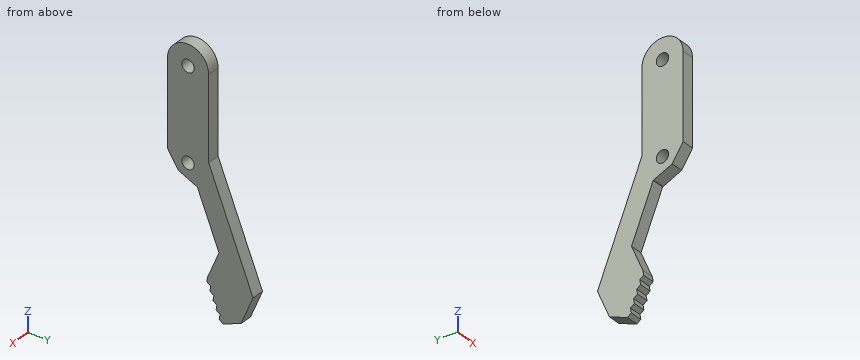
from build123d import *

# Parameters (mm, degrees)
SKETCH1_R             = 5
SKETCH1_R_2           = 1.5
BOSS_EXTRUDE1_DEPTH   = 3
BOSS_EXTRUDE2_START   = -3
BOSS_EXTRUDE2_DEPTH   = 3
CUT_EXTRUDE2_DEPTH    = 65.81382707
CORTAR_EXTRUIR1_DEPTH = 3
SCALE1_SCALE          = 0.888888889


# Read off the part's stored shape, not the designer's step: Cortar-Extruir1
with BuildPart() as part:
    # Sketch1 → Boss-Extrude1 (new body)
    # profile 1 of 3: a face of its own
    with BuildSketch(Plane(origin=(0, 0, 0), x_dir=(0, 0, -1), z_dir=(1, 0, 0))):
        with Locations((5, 5)):
            Circle(SKETCH1_R)
        with Locations((5, 5)):
            Circle(SKETCH1_R_2, mode=Mode.SUBTRACT)
    # profile 2 of 3: a face of its own
    with BuildSketch(Plane(origin=(0, 0, 0), x_dir=(0, 0, -1), z_dir=(1, 0, 0))):
        with BuildLine():
            ThreePointArc((10, 5), (8.535533906, 1.464466094), (5, 0))
            Line((5, 0), (27, 0))
            ThreePointArc((27, 0), (22, 5), (27, 10))
            Line((27, 10), (5, 10))
            ThreePointArc((5, 10), (8.535533906, 8.535533906), (10, 5))
        make_face()
    # profile 3 of 3: a face of its own
    with BuildSketch(Plane(origin=(0, 0, 0), x_dir=(0, 0, -1), z_dir=(1, 0, 0))):
        with Locations((27, 5)):
            Circle(SKETCH1_R)
        with Locations((27, 5)):
            Circle(SKETCH1_R_2, mode=Mode.SUBTRACT)
    extrude(amount=BOSS_EXTRUDE1_DEPTH)

    # Sketch2 → Boss-Extrude2 (add)
    with BuildSketch(Plane(origin=(3, 0, 0), x_dir=(0, 0, -1), z_dir=(1, 0, 0)).offset(BOSS_EXTRUDE2_START)):
        with BuildLine():
            ThreePointArc((27, 10), (29.694507461, 9.21184396), (31.53953799, 7.095851816))
            Line((31.53953799, 7.095851816), (31.610157793, 7.262674791))
            Line((31.610157793, 7.262674791), (44.585599673, 12.519851602))
            Line((44.585599673, 12.519851602), (51.097249205, 9.763328363))
            Line((51.097249205, 9.763328363), (60.365421977, 13.518454657))
            Line((60.365421977, 13.518454657), (56.610295683, 22.786627428))
            Line((56.610295683, 22.786627428), (25.051124858, 10))
            Line((25.051124858, 10), (27, 10))
        make_face()
        Polygon((60.365421977, 13.518454657), (51.097249205, 9.763328363), (51.333822162, 9.179433479), (60.601994933, 12.934559772), align=None)
    extrude(amount=BOSS_EXTRUDE2_DEPTH)

    # Sketch4 → Cut-Extrude2 (cut, through all)
    with BuildSketch(Plane(origin=(3, 0, 0), x_dir=(0, 0, -1), z_dir=(1, 0, 0))):
        Polygon((56.610295683, 22.786627428), (51.684261855, 20.790777803), (58.606145308, 17.8605936), align=None)
    extrude(amount=-CUT_EXTRUDE2_DEPTH, mode=Mode.SUBTRACT)

    # Cortar-Extruir1 outline → Cortar-Extruir1 (cut)
    with BuildSketch(Plane.YZ):
        with BuildLine():
            ThreePointArc((0, -27), (2.305492538, -31.21184396), (7.095851816, -31.53953799))
            Line((7.095851816, -31.53953799), (2.664871714, -29.583874941))
            Line((2.664871714, -29.583874941), (0, -25.53953799))
            Line((0, -25.53953799), (0, -27))
        make_face()
        Polygon((13.518454657, -60.365421977), (12.559047143, -59.675177656), (12.934559772, -60.601994933), align=None)
        Polygon((12.767429398, -58.511787422), (11.808021884, -57.821543102), (12.559047143, -59.675177656), align=None)
        Polygon((12.01640414, -56.658152868), (11.056996626, -55.967908548), (11.808021884, -57.821543102), align=None)
        Polygon((11.265378881, -54.804518314), (10.305971367, -54.114273993), (11.056996626, -55.967908548), align=None)
        Polygon((10.514353622, -52.95088376), (9.554946108, -52.260639439), (10.305971367, -54.114273993), align=None)
        Polygon((9.554946108, -52.260639439), (9.763328363, -51.097249205), (9.179433479, -51.333822162), align=None)
    extrude(amount=CORTAR_EXTRUIR1_DEPTH, mode=Mode.SUBTRACT)


with BuildPart() as part_1:
    # Scale1: scaled about (1.5, 8.912185075, -28.416581742)
    add(part.part.scale(SCALE1_SCALE).moved(Location((0.166666667, 0.990242786, -3.157397971))))


solid = part_1.part
Geometry check sheet. Reference: the model listing, model coordinates, mm. Give positions to 0.01 mm unless a question says otherwise; leave off trailing zeros. Order: outer loops, then holes, each group sorted by start corner. A loop starts at its lowest first (then second) coordinate and runs counter-clockwise, first axis right, second up. Notation, with made-up numbers: M 86,31.25 L 141,31.25 A19 ccw 141,49.25 Z; hole C 82,37.5 d10. An arc over 180 degrees is marked long. Use a Markdown table: item, result.
Item 1: Section check C-C (y = 8.25). Record the cut outline in (x, z).
Answers follow:
| item | result |
|---|---|
| outline | M 0.17,-33.24 L 2.83,-33.24 L 2.83,-4.16 L 0.17,-4.16 Z |
Item 2: Section check A-A (x = 1.9). Record the cut outline in (y, z), and give its area (3 significant figures).
Answers follow:
| item | result |
|---|---|
| outline | M 0.99,-25.86 L 3.36,-29.45 L 7.3,-31.19 L 7.45,-31.26 L 12.12,-42.79 L 9.67,-48.58 L 9.48,-49.61 L 10.34,-50.22 L 10.15,-51.26 L 11,-51.87 L 10.82,-52.91 L 11.67,-53.52 L 11.49,-54.55 L 12.34,-55.17 L 12.15,-56.2 L 13.01,-56.82 L 16.87,-55.25 L 19.47,-49.1 L 9.88,-25.43 L 9.88,-7.6 A4.44 ccw 0.99,-7.6 Z; hole C 5.43,-27.16 d2.67; hole C 5.43,-7.6 d2.67 |
| area | 376 mm2 |
Item 3: Material ranges on line 1 along Z through (x, y) = (1.35, 6.5); line 2 along Y through (x, z) = (2.3, -12.5); line 3 along Z through (x, y) = (1.2, 4.75), recorded low to high.
Answers follow:
| item | result |
|---|---|
| line 1 | z = -30.84 to -27.96, -26.36 to -8.4, -6.8 to -3.29 |
| line 2 | y = 0.99 to 9.88 |
| line 3 | z = -30.07 to -28.3, -26.01 to -8.75, -6.46 to -3.21 |
Item 4: Depth check by flat-ended pin: P1, Ø2.5, axis at y = 5.43, z = -7.6, coming from the -X side; P2, Ø0.8, axis at x = 1, z = -13, coming from the +Y side. Enter the tip coordinate at first touch or a pass-through.
Answers follow:
| item | result |
|---|---|
| P1 | passes through |
| P2 | stops at y = 9.88 |
Item 5: Section check B-B (z = -23). Record the cut outline in (x, y).
Answers follow:
| item | result |
|---|---|
| outline | M 0.17,0.99 L 2.83,0.99 L 2.83,9.88 L 0.17,9.88 Z |
